Read the model definition and answer for the solid it produces. Units are mm, in the model's axes. A direction names the side the tool comes from. Coordinates: 2 decimals unless noted, no trailing zeros. Loops run counter-clockwise (first coordinate to the right, second up) from the corner with the lowest first, then second, coordinate; pieces in that order, holes last.
from build123d import *

# Parameters (mm, degrees)
PAD_DEPTH = 3


with BuildPart() as part:
    # Sketch → Pad (new body)
    with BuildSketch(Plane.XY):
        with BuildLine():
            Line((7, 0), (12.9, 0))
            ThreePointArc((12.9, 0), (14.314214, 0.585786), (14.9, 2))
            Line((14.9, 2), (14.9, 3))
            ThreePointArc((16.9, 5), (15.485786, 4.414214), (14.9, 3))
            Line((16.9, 5), (17, 5))
            ThreePointArc((19, 3), (18.414214, 4.414214), (17, 5))
            Line((19, 3), (19, 2))
            ThreePointArc((19, 2), (19.585786, 0.585786), (21, 0))
            Line((21, 0), (33, 0))
            ThreePointArc((33, 0), (34.414214, 0.585786), (35, 2))
            Line((35, 2), (35, 3))
            ThreePointArc((37, 5), (35.585786, 4.414214), (35, 3))
            Line((37, 5), (38, 5))
            ThreePointArc((38, 5), (39.414214, 5.585786), (40, 7))
            Line((40, 7), (40, 14))
            ThreePointArc((40, 14), (39.414214, 15.414214), (38, 16))
            Line((38, 16), (7, 16))
            ThreePointArc((7, 16), (5.585786, 15.414214), (5, 14))
            Line((5, 14), (5, 13))
            ThreePointArc((3, 11), (4.414214, 11.585786), (5, 13))
            Line((3, 11), (2, 11))
            ThreePointArc((2, 11), (0.585786, 10.414214), (0, 9))
            Line((0, 9), (0, 7))
            ThreePointArc((0, 7), (0.585786, 5.585786), (2, 5))
            Line((3, 5), (2, 5))
            ThreePointArc((5, 3), (4.414214, 4.414214), (3, 5))
            Line((5, 2), (5, 3))
            ThreePointArc((5, 2), (5.585786, 0.585786), (7, 0))
        make_face()
        with BuildLine():
            ThreePointArc((21.9, 11.05), (19.85, 9), (21.9, 6.95))
            Line((21.9, 6.95), (30.9, 6.95))
            ThreePointArc((30.9, 6.95), (32.95, 9), (30.9, 11.05))
            Line((21.9, 11.05), (30.9, 11.05))
        make_face(mode=Mode.SUBTRACT)
        with BuildLine():
            ThreePointArc((13.05, 12), (11, 14.05), (8.95, 12))
            Line((8.95, 12), (8.95, 4))
            ThreePointArc((8.95, 4), (11, 1.95), (13.05, 4))
            Line((13.05, 12), (13.05, 4))
        make_face(mode=Mode.SUBTRACT)
    extrude(amount=PAD_DEPTH)


solid = part.part
Q1. A cutting plane is placed at B-B (y = 6.5). Give the vertices of the cut face in (x, z).
Findings below:
outline: (0.06, 0) - (8.95, 0) - (8.95, 3) - (0.06, 3) - close; (13.05, 0) - (39.94, 0) - (39.94, 3) - (13.05, 3) - close
Q2. A cutting plane is placed at D-D (y = 15.25). Give the vertices of the cut face in (x, z).
Findings below:
outline: (5.44, 0) - (39.56, 0) - (39.56, 3) - (5.44, 3) - close
Q3. Flat-ended cylindrical pins translate along their axes: pin 1 Ø0.8 at (y, z) = (13.5, 1) entering from -X; pin 2 Ø3 at (x, y) = (7.5, 9.5) entering from -Z; pin 3 Ø1.1 at (x, z) = (37.5, 1.5) entering from -Y; pin 4 Ø0.8 at (y, z) = (2.5, 2) entering from +X. Find the tip coordinate at first contact, or state that the pin passes through.
Findings below:
pin 1: stops at x = 5
pin 2: stops at z = 0
pin 3: stops at y = 5
pin 4: stops at x = 35
Q4. Determine the mould class of faces 6 (the face through (11.05, 14.05, 1.48)), 7 (the face through (5, 2.5, 1.5)), 8 (the face through (4.4, 11.57, 1.48)) for opening direction Y: +Y half, -Y half, draft (parallel to the pull), parting line (faces both ways), or undercut.
Findings below:
face 6: undercut
face 7: draft
face 8: +Y half
Q5. Straight lines are drawn through the part: probe 1 along X at (y, z) = (10.75, 2.45); probe 2 along X at (y, z) = (7.5, 1.25); probe 3 along Y at (x, z) = (29, 0.8). For each, find the intervals that lie inside material, in ascending order.
Findings below:
probe 1: x = 1.03 to 8.95, 13.05 to 20.83, 31.97 to 40
probe 2: x = 0 to 8.95, 13.05 to 20.5, 32.3 to 40
probe 3: y = 0 to 6.95, 11.05 to 16
Q6. Which of the six approach directions +Z, -Z, +X, -X, +Y, -Y give full straight-line access (tool end or side, diameter ignored) to faces 1 (the face through (27, 0, 1)), 2 (the face through (2.5, 11, 1.5)), 3 (the face through (19.85, 9.05, 1.48)), 4 (the face through (19.57, 0.6, 1.48)), 5 (the face through (40, 10, 1))?
Findings below:
face 1: +Z, -Z, +X, -X, -Y
face 2: +Z, -Z, -X, +Y
face 3: +Z, -Z
face 4: +Z, -Z, -Y
face 5: +Z, -Z, +X, +Y, -Y
Q7. A cutting plane is placed at A-A (x = 11). Give the vertices of the cut face in (y, z), then the cut area to 3 significant figures.
Findings below:
outline: (0, 0) - (1.95, 0) - (1.95, 3) - (0, 3) - close; (14.05, 0) - (16, 0) - (16, 3) - (14.05, 3) - close
area: 11.7 mm2
Q8. A cutting plane is placed at C-C (z = 1.95). Count the separate pieces of the cut face and the enclosed holes in it, then the cut area to 3 significant figures.
Findings below:
separate pieces: 1
enclosed holes: 2
area: 445 mm2
